```python
from build123d import *

# Parameters (mm, degrees)
F1_DEPTH = 15
F2_DEPTH = 20
F3_DEPTH = 35
F5_R     = 5.08
F6_R     = 5.08
F7_R     = 5.08
F8_R     = 5.08
F9_R     = 5.08
F10_D    = 7.5


with BuildPart() as f1:
    # F0 (on Front) → F1 (new body)
    with BuildSketch(Plane.XZ):
        with BuildLine():
            add(Edge.make_bspline(
                [(-9.0078394144, -14.6261555421), (-14.006421456, -12.219431046), (-21.4777151753, -8.7987738685), (-25.373944364, -2.1621207849), (-26.2406452466, 0)],
                knots=[0, 0, 0, 0, 0.4219290451, 0.6690640109, 0.6690640109, 0.6690640109, 0.6690640109], degree=3))
            Line((-9.0078394144, -14.6261555421), (35.9921605856, -14.6261555421))
            add(Edge.make_bspline(
                [(35.9921605856, -14.6261555421), (40.7291624411, -12.3453770516), (49.6848707909, -7.8887732182), (53.4571237511, -0.6658874553), (53.9921605856, 2.4431246054)],
                knots=[0, 0, 0, 0, 0.3998491278, 0.7291996551, 0.7291996551, 0.7291996551, 0.7291996551], degree=3))
            add(Edge.make_bspline(
                [(53.9921605856, 2.4431246054), (54.4320814217, 4.9994330631), (54.0818703156, 7.4521168259), (53.8528075786, 9.4431246054)],
                knots=[0.7291996551, 0.7291996551, 0.7291996551, 0.7291996551, 1, 1, 1, 1], degree=3))
            Line((53.8528075786, 9.4431246054), (45.8528075786, 9.4431246054))
            add(Edge.make_bspline(
                [(45.8528075786, 9.4431246054), (45.9380271862, 8.8438899514), (46.0685244466, 6.2436364853), (46.6196397936, -1.8447716738), (39.5795212377, -5.0875957452), (35.9921605856, -6.6261555421)],
                knots=[0, 0, 0, 0, 0.2232213361, 0.5705276676, 1, 1, 1, 1], degree=3))
            Line((35.9921605856, -6.6261555421), (-9.0078394144, -6.6261555421))
            add(Edge.make_bspline(
                [(-19.0078394144, 7), (-19.053505059, 6.7049076197), (-19.5120334536, 6.7583982823), (-19.2237277553, -2.712889397), (-13.0753368013, -4.8592315184), (-9.0078394144, -6.6261555421)],
                knots=[0, 0, 0, 0, 0.1097832683, 0.5084327524, 1, 1, 1, 1], degree=3))
            Line((-19.0078394144, 7), (-27.0078394144, 7))
            add(Edge.make_bspline(
                [(-26.2406452466, 0), (-26.592756236, 0.8783958848), (-27.4419103236, 3.6162903723), (-27.2028414979, 5.3050465987), (-27.0078394144, 7)],
                knots=[0.6690640109, 0.6690640109, 0.6690640109, 0.6690640109, 0.7694665132, 1, 1, 1, 1], degree=3))
        make_face()
    extrude(amount=-F1_DEPTH)

    # F0 (on Front) → F2 (join)
    with BuildSketch(Plane.XZ):
        with BuildLine():
            add(Edge.make_bspline(
                [(-9.0078394144, -14.6261555421), (-14.006421456, -12.219431046), (-21.4777151753, -8.7987738685), (-25.373944364, -2.1621207849), (-26.2406452466, 0)],
                knots=[0, 0, 0, 0, 0.4219290451, 0.6690640109, 0.6690640109, 0.6690640109, 0.6690640109], degree=3))
            Line((-9.0078394144, -14.6261555421), (35.9921605856, -14.6261555421))
            add(Edge.make_bspline(
                [(35.9921605856, -14.6261555421), (40.7291624411, -12.3453770516), (49.6848707909, -7.8887732182), (53.4571237511, -0.6658874553), (53.9921605856, 2.4431246054)],
                knots=[0, 0, 0, 0, 0.3998491278, 0.7291996551, 0.7291996551, 0.7291996551, 0.7291996551], degree=3))
            add(Edge.make_bspline(
                [(53.9921605856, 2.4431246054), (54.4320814217, 4.9994330631), (54.0818703156, 7.4521168259), (53.8528075786, 9.4431246054)],
                knots=[0.7291996551, 0.7291996551, 0.7291996551, 0.7291996551, 1, 1, 1, 1], degree=3))
            Line((53.8528075786, 9.4431246054), (45.8528075786, 9.4431246054))
            add(Edge.make_bspline(
                [(45.8528075786, 9.4431246054), (45.9380271862, 8.8438899514), (46.0685244466, 6.2436364853), (46.6196397936, -1.8447716738), (39.5795212377, -5.0875957452), (35.9921605856, -6.6261555421)],
                knots=[0, 0, 0, 0, 0.2232213361, 0.5705276676, 1, 1, 1, 1], degree=3))
            Line((35.9921605856, -6.6261555421), (-9.0078394144, -6.6261555421))
            add(Edge.make_bspline(
                [(-19.0078394144, 7), (-19.053505059, 6.7049076197), (-19.5120334536, 6.7583982823), (-19.2237277553, -2.712889397), (-13.0753368013, -4.8592315184), (-9.0078394144, -6.6261555421)],
                knots=[0, 0, 0, 0, 0.1097832683, 0.5084327524, 1, 1, 1, 1], degree=3))
            Line((-19.0078394144, 7), (-27.0078394144, 7))
            add(Edge.make_bspline(
                [(-26.2406452466, 0), (-26.592756236, 0.8783958848), (-27.4419103236, 3.6162903723), (-27.2028414979, 5.3050465987), (-27.0078394144, 7)],
                knots=[0.6690640109, 0.6690640109, 0.6690640109, 0.6690640109, 0.7694665132, 1, 1, 1, 1], degree=3))
        make_face()
        with BuildLine():
            Line((-54.9591742456, 0), (-26.2406452466, 0))
            add(Edge.make_bspline(
                [(-26.2406452466, 0), (-26.592756236, 0.8783958848), (-27.4419103236, 3.6162903723), (-27.2028414979, 5.3050465987), (-27.0078394144, 7)],
                knots=[0.6690640109, 0.6690640109, 0.6690640109, 0.6690640109, 0.7694665132, 1, 1, 1, 1], degree=3))
            Line((-27.0078394144, 7), (-54.9591742456, 7))
            Line((-54.9591742456, 7), (-54.9591742456, 0))
        make_face()
        with BuildLine():
            add(Edge.make_bspline(
                [(53.9921605856, 2.4431246054), (54.4320814217, 4.9994330631), (54.0818703156, 7.4521168259), (53.8528075786, 9.4431246054)],
                knots=[0.7291996551, 0.7291996551, 0.7291996551, 0.7291996551, 1, 1, 1, 1], degree=3))
            Line((53.9921605856, 2.4431246054), (83.8528075786, 2.4431246054))
            Line((83.8528075786, 2.4431246054), (83.8528075786, 9.4431246054))
            Line((83.8528075786, 9.4431246054), (53.8528075786, 9.4431246054))
        make_face()
    extrude(amount=F2_DEPTH)

    # F0 (on Front) → F3 (join)
    with BuildSketch(Plane.XZ):
        with BuildLine():
            add(Edge.make_bspline(
                [(-9.0078394144, -14.6261555421), (-14.006421456, -12.219431046), (-21.4777151753, -8.7987738685), (-25.373944364, -2.1621207849), (-26.2406452466, 0)],
                knots=[0, 0, 0, 0, 0.4219290451, 0.6690640109, 0.6690640109, 0.6690640109, 0.6690640109], degree=3))
            Line((-9.0078394144, -14.6261555421), (35.9921605856, -14.6261555421))
            add(Edge.make_bspline(
                [(35.9921605856, -14.6261555421), (40.7291624411, -12.3453770516), (49.6848707909, -7.8887732182), (53.4571237511, -0.6658874553), (53.9921605856, 2.4431246054)],
                knots=[0, 0, 0, 0, 0.3998491278, 0.7291996551, 0.7291996551, 0.7291996551, 0.7291996551], degree=3))
            add(Edge.make_bspline(
                [(53.9921605856, 2.4431246054), (54.4320814217, 4.9994330631), (54.0818703156, 7.4521168259), (53.8528075786, 9.4431246054)],
                knots=[0.7291996551, 0.7291996551, 0.7291996551, 0.7291996551, 1, 1, 1, 1], degree=3))
            Line((53.8528075786, 9.4431246054), (45.8528075786, 9.4431246054))
            add(Edge.make_bspline(
                [(45.8528075786, 9.4431246054), (45.9380271862, 8.8438899514), (46.0685244466, 6.2436364853), (46.6196397936, -1.8447716738), (39.5795212377, -5.0875957452), (35.9921605856, -6.6261555421)],
                knots=[0, 0, 0, 0, 0.2232213361, 0.5705276676, 1, 1, 1, 1], degree=3))
            Line((35.9921605856, -6.6261555421), (-9.0078394144, -6.6261555421))
            add(Edge.make_bspline(
                [(-19.0078394144, 7), (-19.053505059, 6.7049076197), (-19.5120334536, 6.7583982823), (-19.2237277553, -2.712889397), (-13.0753368013, -4.8592315184), (-9.0078394144, -6.6261555421)],
                knots=[0, 0, 0, 0, 0.1097832683, 0.5084327524, 1, 1, 1, 1], degree=3))
            Line((-19.0078394144, 7), (-27.0078394144, 7))
            add(Edge.make_bspline(
                [(-26.2406452466, 0), (-26.592756236, 0.8783958848), (-27.4419103236, 3.6162903723), (-27.2028414979, 5.3050465987), (-27.0078394144, 7)],
                knots=[0.6690640109, 0.6690640109, 0.6690640109, 0.6690640109, 0.7694665132, 1, 1, 1, 1], degree=3))
        make_face()
    extrude(amount=F3_DEPTH)

    # F5
    f5_edges = [f1.edges().sort_by_distance(p)[0] for p in [
        (83.852808, -10, 9.443125),
    ]]
    fillet(f5_edges, radius=F5_R)

    # F6
    f6_edges = [f1.edges().sort_by_distance(p)[0] for p in [
        (-54.959174, -10, 7),
        (49.852808, -35, 9.443125),
    ]]
    fillet(f6_edges, radius=F6_R)

    # F7
    f7_edges = [f1.edges().sort_by_distance(p)[0] for p in [
        (-23.007839, -35, 7),
    ]]
    fillet(f7_edges, radius=F7_R)

    # F8
    f8_edges = [f1.edges().sort_by_distance(p)[0] for p in [
        (-23.007839, 15, 7),
    ]]
    fillet(f8_edges, radius=F8_R)

    # F9
    f9_edges = [f1.edges().sort_by_distance(p)[0] for p in [
        (49.852808, 15, 9.443125),
    ]]
    fillet(f9_edges, radius=F9_R)

    # F10 (through all)
    with Locations(Plane(origin=(0, 0, 0), x_dir=(1, 0, 0), z_dir=(0, 0, -1))):
        with Locations((-44.82346192, 7.6027605683), (74.7854933143, 14.3004301935)):
            Hole(F10_D / 2)


solid = f1.part
```
Part model, mm, in its own coordinate system. A direction names the side the tool comes from. Round coordinates to 2 decimals unless told otherwise and drop trailing zeros. Loops run counter-clockwise (first coordinate to the right, second up) from the corner with the lowest first, then second, coordinate; pieces in that order, holes last. Notation, with made-up numbers: (-3, -5) -> (50, -5) arc R15 cw to (50, 8) -> close; hole circle Ø1 at (66, -11.75). An arc over 180 degrees is marked (long way). Use a Markdown table: item, result.
1) Cut at C-C, the plane x = 66.5. List the corners of the cut face in (y, z), and give its area (3 significant figures).
The answers:
| item | result |
|---|---|
| outline | (-20, 2.44) -> (0, 2.44) -> (0, 9.44) -> (-20, 9.44) -> close |
| area | 140 mm2 |
2) Probe line 1 (Y direction, x = -40.5, z = 4); line 2 (X direction, y = -6, z = 3); line 3 (X direction, y = -16, z = 5). List the from-to ranges inside material, lowest first. Write a range as [from, to].
The answers:
| item | result |
|---|---|
| line 1 | y = [-20, 0] |
| line 2 | x = [-54.84, -48.21], [-41.43, -19.15], [46.11, 83.85] |
| line 3 | x = [-53.92, -19.33], [46.14, 71.44], [78.13, 83.81] |
3) Tool access for faces 1 (the flat face through (-41, -10, 0)), 2 (the flat face through (69, -10, 2.443)), 3 (the cylindrical face through (-23.139, -33.551, 5.472)): list every direction of +Z, -Z, +X, -X, +Y, -Y with a clear straight run to the whole face (end or side of a thin tool).
The answers:
| item | result |
|---|---|
| face 1 | -Z, -X, +Y, -Y |
| face 2 | -Z, +X, +Y, -Y |
| face 3 | +Z, -X, -Y |
4) Pull direction X, two halves, no side cores. Call faces 4 (the cylindrical face through (78.53, -14.47, 5.99)), 5 (the cylindrical face through (-53.432, -10.14, 5.551)), 6 (the flat face through (-31, -10, 7)): pulls with the +X half, pulls with the -X half, needs draft (parallel to the pull), parting line crosses it, or undercut.
The answers:
| item | result |
|---|---|
| face 4 | undercut |
| face 5 | pulls with the -X half |
| face 6 | needs draft |
5) Drop flat-ended pins along their axis: pin 1 Ø22.5 at (x, y) = (22, -4) entering from +Z; pin 2 Ø6 at (x, y) = (68.5, -14.5) entering from -Z; pin 3 Ø2 at (x, z) = (-38.5, 3) entering from -Y. Give the stop position or say it passes through.
The answers:
| item | result |
|---|---|
| pin 1 | stops at z = -6.63 |
| pin 2 | stops at z = 2.44 |
| pin 3 | stops at y = -20 |
6) Cut at B-B, the plane x = 30.5. List the corners of the cut face in (y, z), and give its area (3 significant figures).
The answers:
| item | result |
|---|---|
| outline | (-35, -14.63) -> (15, -14.63) -> (15, -6.63) -> (-35, -6.63) -> close |
| area | 400 mm2 |
7) Cut at A-A, the plane x = -44.5. List the corners of the cut face in (y, z).
The answers:
| item | result |
|---|---|
| outline | (-20, 0) -> (-11.34, 0) -> (-11.34, 7) -> (-20, 7) -> close; (-3.87, 0) -> (0, 0) -> (0, 7) -> (-3.87, 7) -> close |
